The listing builds one solid part. Answer for the finished solid, in the listing's coordinates (mm). Give positions to 0.01 mm unless a question says otherwise; leave off trailing zeros. Write each loop counter-clockwise with the first axis right and the second up, starting at its lowest first coordinate (ties: lowest second). Pieces come first, ordered by that corner, then holes. Notation, with made-up numbers: (18.25, 60) -> (28.25, 60) arc R19 cw to (28.25, 93) -> close; hole circle Ø11 at (-21, 60.25). An arc over 180 degrees is marked (long way). Put each result on its own line as item: value. Start each with the question number.
1) Find the intervals of material crossed by line 1 along X through (y, z) = (100, -6.75); line 2 along Y through (x, z) = (85, -4.5); line 3 along Y through (x, z) = (188.5, -0.5), in increasing order. Write a range as from..to.
2) A cutting plane is placed at A-A (x = 185). Write down the section's boundary in (y, z), then the cut area to 3 significant figures.
3) A cutting plane is placed at C-C (z = -4.75). Write down the section's boundary in (x, y).
4) A cutting plane is placed at B-B (y = 100). Write down the section's boundary in (x, z).
5) For a pull along X with two mould halves and no side action, classify faces 1 (the flat face through (0, 114, -5)), 2 (the flat face through (133, 0, -5)), 3 (the cylindrical face through (173, 109, -5)), 4 (the cylindrical face through (81.748, 114.643, -4.93)) as released by +X, released by -X, zero draft, split by the parting line, or undercut.
from build123d import *

# Parameters (mm, degrees)
BOSS_EXTRUDE1_DEPTH = 10


with BuildPart() as part:
    # Sketch1 → Boss-Extrude1 (new body)
    with BuildSketch(Plane.XY):
        with BuildLine():
            Line((0, 175), (0, 100))
            Line((0, 100), (70, 100))
            ThreePointArc((70, 100), (85, 115), (100, 100))
            Line((100, 100), (170, 100))
            ThreePointArc((170, 100), (185, 115), (200, 100))
            Line((200, 100), (270, 100))
            Line((270, 100), (270, 225))
            Line((270, 225), (0, 225))
            Line((0, 225), (0, 175))
        make_face()
        with BuildLine():
            Line((0, 100), (0, 0))
            Line((0, 0), (270, 0))
            Line((270, 0), (270, 100))
            Line((270, 100), (200, 100))
            ThreePointArc((200, 100), (185, 85), (170, 100))
            Line((170, 100), (100, 100))
            ThreePointArc((100, 100), (85, 85), (70, 100))
            Line((70, 100), (0, 100))
        make_face()
    extrude(amount=-BOSS_EXTRUDE1_DEPTH)


solid = part.part
Reply:
1. line 1: x = 0..70, 100..170, 200..270
1. line 2: y = 0..85, 115..225
1. line 3: y = 0..85.41, 114.59..225
2. outline: (0, -10) -> (85, -10) -> (85, 0) -> (0, 0) -> close; (115, -10) -> (225, -10) -> (225, 0) -> (115, 0) -> close
2. area: 1,950 mm2
3. outline: (0, 0) -> (270, 0) -> (270, 225) -> (0, 225) -> close; hole circle Ø30 at (85, 100); hole circle Ø30 at (185, 100)
4. outline: (0, -10) -> (70, -10) -> (70, 0) -> (0, 0) -> close; (100, -10) -> (170, -10) -> (170, 0) -> (100, 0) -> close; (200, -10) -> (270, -10) -> (270, 0) -> (200, 0) -> close
5. face 1: released by -X
5. face 2: zero draft
5. face 3: undercut
5. face 4: undercut
